Input: dimensioned drawing with shaded views. Units: mm. Origin: part minimum x, y, z. Round coordinates to 2 decimals unless told otherwise and drop trailing zeros. Order: outer loops, then holes, each group sorted by start corner. A loop starts at its lowest first (then second) coordinate and runs counter-clockwise, first axis right, second up. Notation, with made-up numbers: (16, 50) - (23, 50) arc R30 cw to (23, 87) - close; hole circle Ø1 at (17, 74). An arc over 180 degrees is marked (long way). Return JSON: item names as keys, results as strings. Group by question number.
1) Section B-B, the plane x = 35.5. Return loops of the section in (y, z) (1 decimal).
2) Contact query for flat-ended pins moving along their axis: P1, Ø8, axis at x = 210.5, z = 32, coming from the -Y side; P2, Ø10, axis at x = 71.5, z = 21.5, coming from the +Y side; P3, Ø4, axis at x = 72, y = 136, coming from the +Z side; P4, Ø10, axis at x = 144, z = 19.5, coming from the -Y side (1 decimal). Output: stop coordinate, or through.
3) Ray query, line 1 (Y direction, x = 74, z = 24) (1 decimal); line 2 (Z direction, x = 214, y = 27); line 3 (Y direction, x = 143.5, z = 55). Return the intervals inside material, ascending. Write a range as from..to.
4) Mould query, pull axis Y, two halves, no side actions, for the marked faces 1 and 2. Classes: pulls with the +Y half, pulls with the -Y half, needs draft (parallel to the pull), parting line crosses it, or undercut.
5) Section A-A, the plane z = 22. Return loops of the section in (x, y) (1 decimal).
6) Section C-C, the plane y = 55.5. Return loops of the section in (x, z) (1 decimal), plus the area to 3 significant figures.
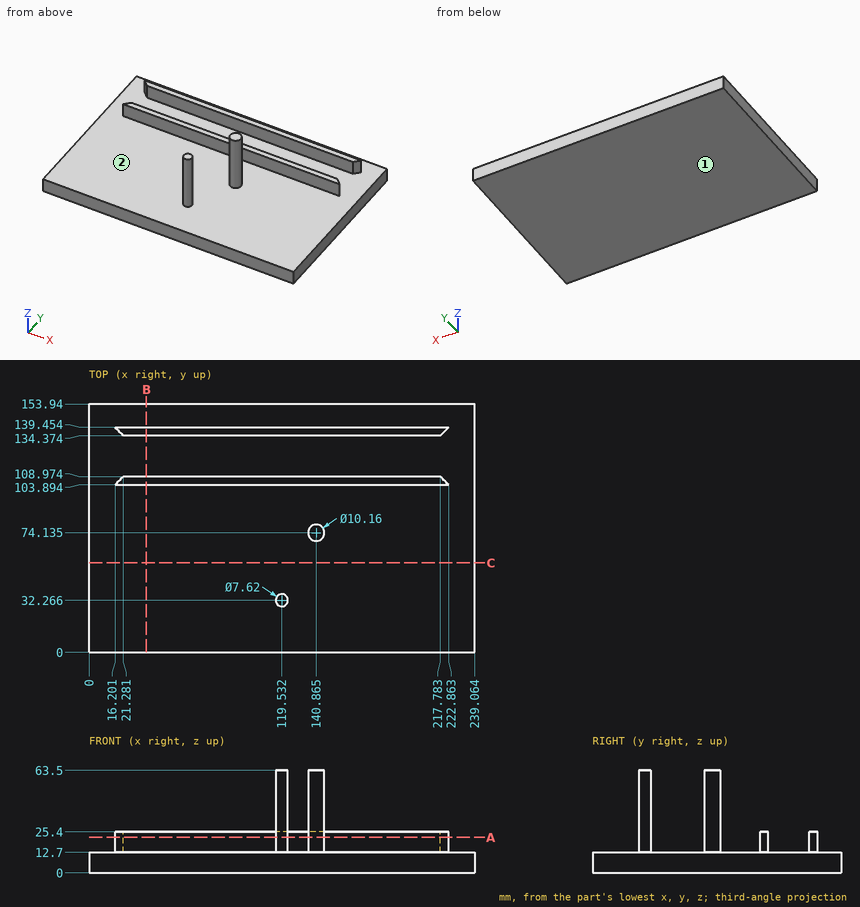
Geometry check:
{
 "1": {"outline": "(0, 0) - (153.9, 0) - (153.9, 12.7) - (139.5, 12.7) - (139.5, 25.4) - (134.4, 25.4) - (134.4, 12.7) - (109, 12.7) - (109, 25.4) - (103.9, 25.4) - (103.9, 12.7) - (0, 12.7) - close"},
 "2": {"P1": "through", "P2": "y = 139.45", "P3": "z = 25.4", "P4": "y = 69.1"},
 "3": {"line 1": "103.9..109, 134.4..139.5", "line 2": "0..12.7", "line 3": "69.79..78.48"},
 "4": {"face 1": "needs draft", "face 2": "undercut"},
 "5": {"outline": "(16.2, 103.9) - (222.9, 103.9) - (217.8, 109) - (21.3, 109) - close; (16.2, 139.5) - (21.3, 134.4) - (217.8, 134.4) - (222.9, 139.5) - close; circle Ø7.6 at (119.5, 32.3); circle Ø10.2 at (140.9, 74.1)"},
 "6": {"outline": "(0, 0) - (239.1, 0) - (239.1, 12.7) - (0, 12.7) - close", "area": "3,040 mm2"}
}
